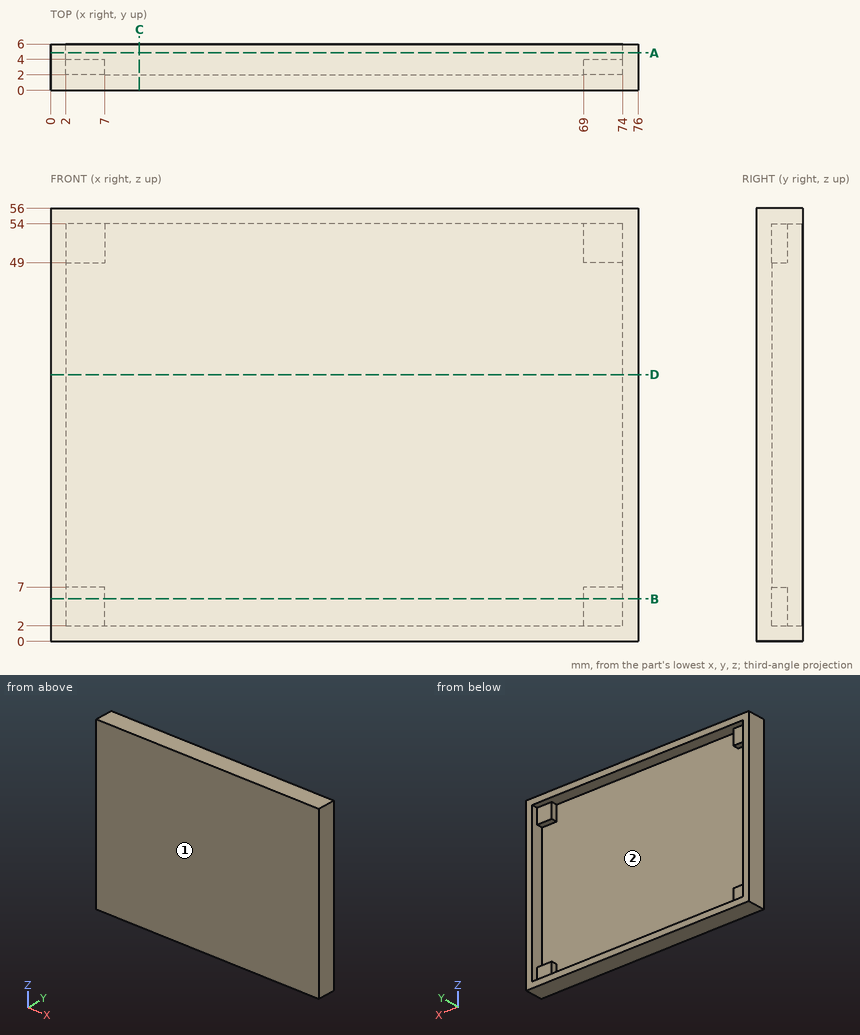
Input: dimensioned drawing with shaded views. Units: mm. Origin: part minimum x, y, z. Coordinates: 2 decimals unless noted, no trailing zeros. Order: outer loops, then holes, each group sorted by start corner. A loop starts at its lowest first (then second) coordinate and runs counter-clockwise, first axis right, second up.
Item 1: Draft query along X for the marked faces 1 and 2. Return one class per face: released by +X, released by -X, zero draft, split by the parting line, or undercut.
Answer:
face 1: zero draft
face 2: undercut
Item 2: Section query D-D (z = 34.5). Output: boundary loops of the cut face in (x, y).
Answer:
outline: (0, 0) - (76, 0) - (76, 6) - (74, 6) - (74, 2) - (2, 2) - (2, 6) - (0, 6) - close
Item 3: Section query A-A (y = 4.85). Output: boundary loops of the cut face in (x, z).
Answer:
outline: (0, 0) - (76, 0) - (76, 56) - (0, 56) - close; hole (2, 2) - (74, 2) - (74, 54) - (2, 54) - close
Item 4: Contact query for flat-ended pins moving along their axis: P1, Ø5.5, axis at x = 4, z = 51.5, coming from the +Y side; P2, Ø4, axis at x = 32.5, z = 38, coming from the +Y side; P3, Ø2.5, axis at x = 72, z = 5.5, coming from the +Y side. Output: stop coordinate, or through.
Answer:
P1: stops at y = 6
P2: stops at y = 2
P3: stops at y = 4
Item 5: Material intervals for line 1 along X through (y, z) = (5.5, 28); line 2 along Z through (x, y) = (65, 4.35); line 3 along Z through (x, y) = (3.5, 2.65), sorted ascending.
Answer:
line 1: x = 0 to 2, 74 to 76
line 2: z = 0 to 2, 54 to 56
line 3: z = 0 to 7, 49 to 56
Item 6: Section query B-B (z = 5.5). Output: boundary loops of the cut face in (x, y), then the cut area to 3 significant figures.
Answer:
outline: (0, 0) - (76, 0) - (76, 6) - (74, 6) - (74, 4) - (69, 4) - (69, 2) - (7, 2) - (7, 4) - (2, 4) - (2, 6) - (0, 6) - close
area: 188 mm2
Item 7: Section query C-C (x = 11.5). Output: boundary loops of the cut face in (y, z).
Answer:
outline: (0, 0) - (6, 0) - (6, 2) - (2, 2) - (2, 54) - (6, 54) - (6, 56) - (0, 56) - close
